Model file for the job. Use its own axes, mm. A direction names the side the tool comes from. Coordinates: 2 decimals unless noted, no trailing zeros. Order: outer loops, then holes, each group sorted by start corner. A loop starts at its lowest first (then second) coordinate and runs counter-clockwise, first axis right, second up. Notation, with made-up numbers: (45, 56) -> (64, 56) arc R22 ccw to (64, 76) -> close; hole circle Ø7 at (89, 12). An arc over 180 degrees is marked (long way). Return JSON: item names as keys, results as strings. Group by question number.
1) Cut at A-A (z = -6.5). Write the cut outline in (x, y), and give its area (3 significant figures).
2) Cut at C-C (z = -12.5). Write the cut outline in (x, y).
3) Which spindle directions (+Z, -Z, +X, -X, +Y, -Y) get a long thin tool onto all of the face, cutting with end or side? Do faces 5 (the flat face through (-6.5, 0, -7)), 6 (the flat face through (0, -6.5, -5)), 7 (the flat face through (6, 0.4, -12)). Say none if no direction does.
4) Flat gauge pins, fed straight in: pin 1 (6.5 mm diameter, centred on x = -10, y = 0, fed in from +Z); pin 2 (7 mm diameter, centred on y = -0.5, z = -10, fed in from +X); pin 3 (2 mm diameter, centred on y = 1, z = -10.5, fed in from -X). Where does each tip first touch, or does it go through?
5) Cut at D-D (y = 1.5). Write the cut outline in (x, z), and give its area (3 significant figures).
6) Cut at B-B (x = -10). Write the cut outline in (y, z).
7) Probe line 1 (X direction, y = 0, z = -15.85); line 2 (Y direction, x = 10, z = -16.1); line 3 (X direction, y = -3.75, z = -11.5). List the from-to ranges inside material, lowest first.
8) Pull direction Y, two halves, no side cores. Call faces 1 (the flat face through (-6, 0, -10)), 2 (the flat face through (-6, 0.4, -12)), 3 (the flat face through (0, 7.5, -9)), 4 (the flat face through (0.4, -2.6, -11.3)): +Y half, -Y half, draft (parallel to the pull), parting line (faces both ways), or undercut.
from build123d import *

# Parameters (mm, degrees)
F1_W      = 13
F1_H      = 15
F2_DEPTH  = 18
F0_W      = 11
F0_H      = 13
F3_DEPTH  = 13
F4_W      = 0.8
F4_H      = 13
F5_DEPTH  = 2
F7_W      = 5.064733
F7_H      = 2.673392
F6_W      = 5.1
F6_H      = 2.730513
F8_DEPTH  = 15
F9_W      = 1.5
F9_H      = 3
F10_DEPTH = 25
F13_W     = 15
F13_H     = 4
F14_DEPTH = 7
F15_R     = 2
F16_DEPTH = 25
F19_DEPTH = 25


with BuildPart() as f2:
    # F1 (on Top) → F2 (new body)
    with BuildSketch(Plane.XY):
        Rectangle(F1_W, F1_H)
    extrude(amount=-F2_DEPTH)

    # F0 (on Top) → F3 (cut)
    with BuildSketch(Plane.XY):
        Rectangle(F0_W, F0_H)
    extrude(amount=-F3_DEPTH, mode=Mode.SUBTRACT)

    # F4 (on face) → F5 (join)
    with BuildSketch(Plane.XY.offset(-13)):
        Rectangle(F4_W, F4_H)
    extrude(amount=F5_DEPTH)

    # F7 (on face) + F6 (on face) → F8 (cut)
    with BuildSketch(Plane.XY.offset(-13)):
        with Locations((-2.967633, -6.836696)):
            Rectangle(F7_W, F7_H)
    with BuildSketch(Plane.XY.offset(-13)):
        with Locations((2.95, -6.865257)):
            Rectangle(F6_W, F6_H)
    extrude(amount=F8_DEPTH, mode=Mode.SUBTRACT)

    # F9 (on face) → F10 (cut)
    with BuildSketch(Plane.YZ.offset(-5.5)):
        with Locations((-0.35, -11.5)):
            Rectangle(F9_W, F9_H)
    extrude(amount=-F10_DEPTH, mode=Mode.SUBTRACT)

    # F11: F2 across plane


with BuildPart() as f2_1:
    add(f2.part)
    add(f2.part.mirror(Plane.YZ), mode=Mode.INTERSECT)

    # F13 (on face) → F14 (join)
    with BuildSketch(Plane(origin=(-6.5, 0, 0), x_dir=(0, -1, 0), z_dir=(-1, 0, 0))):
        with Locations((0, -16)):
            Rectangle(F13_W, F13_H)
    extrude(amount=F14_DEPTH)

    # F15 (on face) → F16 (cut)
    with BuildSketch(Plane.XY.offset(-14)):
        with Locations((-10, 0)):
            Circle(F15_R)
    extrude(amount=-F16_DEPTH, mode=Mode.SUBTRACT)

    # F17: F2 across plane


with BuildPart() as f2_2:
    add(f2_1.part)
    add(f2_1.part.mirror(Plane.YZ))

    # F18 (on face) → F19 (cut)
    with BuildSketch(Plane.XZ.offset(7.5)):
        with BuildLine():
            Line((-13.5, -18), (13.5, -18))
            ThreePointArc((13.5, -18), (0, -14.2), (-13.5, -18))
        make_face()
    extrude(amount=-F19_DEPTH, mode=Mode.SUBTRACT)


solid = f2_2.part
Answers below:
{
 "1": {"outline": "(-6.5, -7.5) -> (-5.5, -7.5) -> (-5.5, 6.5) -> (5.5, 6.5) -> (5.5, -7.5) -> (6.5, -7.5) -> (6.5, 7.5) -> (-6.5, 7.5) -> close; (-0.4, -7.5) -> (0.4, -7.5) -> (0.4, -6.5) -> (-0.4, -6.5) -> close", "area": "41.8 mm^2"},
 "2": {"outline": "(-6.5, -7.5) -> (-5.5, -7.5) -> (-5.5, -1.1) -> (-6.5, -1.1) -> close; (-6.5, 0.4) -> (-5.5, 0.4) -> (-5.5, 6.5) -> (-0.4, 6.5) -> (-0.4, -7.5) -> (0.4, -7.5) -> (0.4, 6.5) -> (5.5, 6.5) -> (5.5, 0.4) -> (6.5, 0.4) -> (6.5, 7.5) -> (-6.5, 7.5) -> close; (5.5, -7.5) -> (6.5, -7.5) -> (6.5, -1.1) -> (5.5, -1.1) -> close"},
 "3": {"face 5": "+Z, -X, +Y, -Y", "face 6": "+Z", "face 7": "+X"},
 "4": {"pin 1": "stops at z = -14", "pin 2": "stops at x = 6.5", "pin 3": "stops at x = -6.5"},
 "5": {"outline": "(-13.5, -18) arc R25.88 cw to (-11.32, -16.81) -> (-11.32, -14) -> (-13.5, -14) -> close; (-8.68, -15.7) arc R25.88 cw to (8.68, -15.7) -> (8.68, -14) -> (6.5, -14) -> (6.5, 0) -> (5.5, 0) -> (5.5, -13) -> (0.4, -13) -> (0.4, -11) -> (-0.4, -11) -> (-0.4, -13) -> (-5.5, -13) -> (-5.5, 0) -> (-6.5, 0) -> (-6.5, -14) -> (-8.68, -14) -> close; (11.32, -16.81) arc R25.88 cw to (13.5, -18) -> (13.5, -14) -> (11.32, -14) -> close", "area": "67.4 mm^2"},
 "6": {"outline": "(-7.5, -16.21) -> (-2, -16.21) -> (-2, -14) -> (-7.5, -14) -> close; (2, -16.21) -> (7.5, -16.21) -> (7.5, -14) -> (2, -14) -> close"},
 "7": {"line 1": "x = -13.5 to -12, 12 to 13.5", "line 2": "y = -7.5 to -2, 2 to 7.5", "line 3": "x = -6.5 to -5.5, -0.4 to 0.4, 5.5 to 6.5"},
 "8": {"face 1": "undercut", "face 2": "undercut", "face 3": "+Y half", "face 4": "draft"}
}
